Design review of the part built by this model. Coordinates are the model's own, in mm. A direction names the side the tool comes from. Coordinates: 2 decimals unless noted, no trailing zeros. Loops run counter-clockwise (first coordinate to the right, second up) from the corner with the lowest first, then second, coordinate; pieces in that order, holes last. Notation, with made-up numbers: M 32,6.5 L 53,6.5 A25 cw 53,23.5 Z; hole C 30,-11.5 d9. An arc over 180 degrees is marked long. Write item = value, one per line. Start each with the question number.
```python
from build123d import *

# Parameters (mm, degrees)
SKETCH1_R           = 1.6
SKETCH1_W           = 40
SKETCH1_H           = 20
BOSS_EXTRUDE1_DEPTH = 3.5


with BuildPart() as part:
    # Sketch1 → Boss-Extrude1 (new body)
    with BuildSketch(Plane.XY):
        with BuildLine():
            ThreePointArc((-50.044200549, -24.884800983), (-49.571119709, -26.026919161), (-48.429001531, -26.5))
            Line((-48.429001531, -26.5), (45.955799451, -26.5))
            ThreePointArc((45.955799451, -26.5), (48.784226576, -25.328427125), (49.955799451, -22.5))
            Line((49.955799451, -22.5), (49.955799451, 22.5))
            ThreePointArc((49.955799451, 22.5), (48.784226576, 25.328427125), (45.955799451, 26.5))
            Line((45.955799451, 26.5), (-48.429001531, 26.5))
            ThreePointArc((-48.429001531, 26.5), (-49.571119709, 26.026919161), (-50.044200549, 24.884800983))
            Line((-50.044200549, 24.884800983), (-50.044200549, -24.884800983))
        make_face()
        with Locations((-44.044200549, -20.5)):
            Circle(SKETCH1_R, mode=Mode.SUBTRACT)
        with Locations((-14.5, -5)):
            Circle(SKETCH1_R, mode=Mode.SUBTRACT)
        with BuildLine():
            ThreePointArc((12.196121371, -14.531845007), (-0.008459876, -18.999966384), (-12.229764581, -14.57779233))
            ThreePointArc((-12.229764581, -14.57779233), (-12.355671334, -13.169194626), (-10.94707363, -13.043287874))
            ThreePointArc((-10.94707363, -13.043287874), (-0.012222052, -16.999969923), (10.907666432, -13.002177111))
            ThreePointArc((10.907666432, -13.002177111), (12.31672785, -13.122783589), (12.196121371, -14.531845007))
        make_face(mode=Mode.SUBTRACT)
        with Locations((43.955799451, -20.5)):
            Circle(SKETCH1_R, mode=Mode.SUBTRACT)
        with Locations((34.5, -5)):
            Circle(SKETCH1_R, mode=Mode.SUBTRACT)
        with Locations((-14.5, 5)):
            Circle(SKETCH1_R, mode=Mode.SUBTRACT)
        with Locations((-44.044200549, 20.5)):
            Circle(SKETCH1_R, mode=Mode.SUBTRACT)
        with Locations((10, 0)):
            Rectangle(SKETCH1_W, SKETCH1_H, mode=Mode.SUBTRACT)
        with Locations((34.5, 5)):
            Circle(SKETCH1_R, mode=Mode.SUBTRACT)
        with BuildLine():
            ThreePointArc((-10.94707363, 13.043287874), (-12.355671334, 13.169194626), (-12.229764581, 14.57779233))
            ThreePointArc((-12.229764581, 14.57779233), (-0.008459876, 18.999966384), (12.196121371, 14.531845007))
            ThreePointArc((12.196121371, 14.531845007), (12.31672785, 13.122783589), (10.907666432, 13.002177111))
            ThreePointArc((10.907666432, 13.002177111), (-0.012222052, 16.999969923), (-10.94707363, 13.043287874))
        make_face(mode=Mode.SUBTRACT)
        with Locations((43.955799451, 20.5)):
            Circle(SKETCH1_R, mode=Mode.SUBTRACT)
    extrude(amount=BOSS_EXTRUDE1_DEPTH)


solid = part.part
```
(1) Take a section at C-C (x = 5.5). State the section outline as (y, z) points, plus the area to 3 significant figures.
(2) Take a section at B-B (y = 2). State the section outline as (x, z) points.
(3) Mouldability with a two-part tool opening along X and no side actions: class faces 3 (the flat face through (10, 10, 2)), 4 (the flat face through (-50.044, 0, 2)), 5 (the flat face through (-12, 0, 3.5)) as +X half, -X half, draft (parallel to the pull), parting line (faces both ways), or undercut.
(4) To check wall thickness, follow L1, parallel to Y at x = 0, z = 2.35; L2, parallel to Y at x = -14.5, z = 2.8; L3, parallel to X at y = -3, z = 0.8. State the ranges of each line that lie inside material, in increasing order.
(5) Tool access review of faces 1 (the flat face through (-12, 0, 0)), 2 (the cylindrical face through (0, 17, 2)): name each direction out of +Z, -Z, +X, -X, +Y, -Y from which nothing blocks a thin tool from reaching the whole face with its end or side.
(6) Insertion check: pin 1 (4 mm diameter, centred on x = -44.04, y = -20.5, fed in from +Z); pin 2 (1.9 mm diameter, centred on x = 34.5, y = 5, fed in from -Z). Each pin has a flat end and moves straight along its axis. Give the tip position at first contact, or say it passes through.
(7) Take a section at D-D (x = -14.5). State the section outline as (y, z) points.
(8) Take a section at A-A (y = 20.5). State the section outline as (x, z) points.
Results list:
q1.outline = M -26.5,0 L -18.17,0 L -18.17,3.5 L -26.5,3.5 Z; M -16.07,0 L -10,0 L -10,3.5 L -16.07,3.5 Z; M 10,0 L 16.07,0 L 16.07,3.5 L 10,3.5 Z; M 18.17,0 L 26.5,0 L 26.5,3.5 L 18.17,3.5 Z
q1.area = 101 mm^2
q2.outline = M -50.04,0 L -10,0 L -10,3.5 L -50.04,3.5 Z; M 30,0 L 49.96,0 L 49.96,3.5 L 30,3.5 Z
q3.face_3 = undercut
q3.face_4 = -X half
q3.face_5 = draft
q4.L1 = -26.5 to -19, -17 to -10, 10 to 17, 19 to 26.5
q4.L2 = -26.5 to -6.6, -3.4 to 3.4, 6.6 to 26.5
q4.L3 = -50.04 to -10, 30 to 49.96
q5.face_1 = -Z, +X, -X, +Y, -Y
q5.face_2 = +Z, -Z
q6.pin_1 = 3.5
q6.pin_2 = through
q7.outline = M -26.5,0 L -6.6,0 L -6.6,3.5 L -26.5,3.5 Z; M -3.4,0 L 3.4,0 L 3.4,3.5 L -3.4,3.5 Z; M 6.6,0 L 26.5,0 L 26.5,3.5 L 6.6,3.5 Z
q8.outline = M -50.04,0 L -45.64,0 L -45.64,3.5 L -50.04,3.5 Z; M -42.44,0 L 42.36,0 L 42.36,3.5 L -42.44,3.5 Z; M 45.56,0 L 49.96,0 L 49.96,3.5 L 45.56,3.5 Z
